Design review of the part built by this model. Coordinates are the model's own, in mm. A direction names the side the tool comes from. Round coordinates to 2 decimals unless told otherwise and drop trailing zeros. Order: outer loops, then holes, each group sorted by start corner. A loop starts at its lowest first (then second) coordinate and runs counter-clockwise, first axis right, second up. Notation, with made-up numbers: (-3.5, 43.5) - (31.5, 43.5) arc R26 cw to (31.5, 71.5) - close; hole circle Ø10 at (81, 30.5). An arc over 180 degrees is marked (long way). Write item = value, one per line.
from build123d import *

# Parameters (mm, degrees)
SKETCH1_R           = 86.36
SKETCH1_R_2         = 1.7859375
BOSS_EXTRUDE1_DEPTH = 6.35
SKETCH2_W           = 69.85
SKETCH2_H           = 114.3
CUT_EXTRUDE1_DEPTH  = 123.296450071


with BuildPart() as part:
    # Sketch1 → Boss-Extrude1 (new body)
    with BuildSketch(Plane.XY):
        Circle(SKETCH1_R)
        with Locations((0, 79.375)):
            Circle(SKETCH1_R_2, mode=Mode.SUBTRACT)
        with Locations((79.375, 0)):
            Circle(SKETCH1_R_2, mode=Mode.SUBTRACT)
        with Locations((0, -79.375)):
            Circle(SKETCH1_R_2, mode=Mode.SUBTRACT)
        with Locations((-79.375, 0)):
            Circle(SKETCH1_R_2, mode=Mode.SUBTRACT)
    extrude(amount=BOSS_EXTRUDE1_DEPTH)

    # Sketch2 → Cut-Extrude1 (cut, through all)
    with BuildSketch(Plane(origin=(0, 0, 0), x_dir=(-1, 0, 0), z_dir=(0, 0, -1))):
        Rectangle(SKETCH2_W, SKETCH2_H)
    extrude(amount=-CUT_EXTRUDE1_DEPTH, mode=Mode.SUBTRACT)


solid = part.part
1) We need section B-B on z = 1.5. Write out the cut boundary in (x, y) (3 decimals).
Findings:
outline = circle Ø172.72 at (0, 0); hole circle Ø3.572 at (-79.375, 0); hole (-34.925, -57.15) - (34.925, -57.15) - (34.925, 57.15) - (-34.925, 57.15) - close; hole circle Ø3.572 at (0, -79.375); hole circle Ø3.572 at (0, 79.375); hole circle Ø3.572 at (79.375, 0)
2) The part is to be moulded in two halves that separate along Y. For faces 1 (the cylindrical face through (-63.65, 58.37, 3.13)), 2 (the flat face through (37, 1, 6.35)), 3 (the flat face through (0, 57.15, 3)), say which applies: released by +Y, released by -Y, zero draft, split by the parting line, or undercut.
Findings:
face_1 = split by the parting line
face_2 = zero draft
face_3 = undercut
3) We need section C-C on y = -49. Write out the cut boundary in (x, z) (3 decimals).
Findings:
outline = (-71.113, 0) - (-34.925, 0) - (-34.925, 6.35) - (-71.113, 6.35) - close; (34.925, 0) - (71.113, 0) - (71.113, 6.35) - (34.925, 6.35) - close
4) We need section A-A on x = -9. Write out the cut boundary in (y, z), and give its area (3 significant figures).
Findings:
outline = (-85.89, 0) - (-57.15, 0) - (-57.15, 6.35) - (-85.89, 6.35) - close; (57.15, 0) - (85.89, 0) - (85.89, 6.35) - (57.15, 6.35) - close
area = 365 mm^2
5) For faces 4 (the flat face through (-34.925, -1, 3)), 5 (the flat face through (37, 1, 0)), list the 3-axis set-ups (+Z, -Z, +X, -X, +Y, -Y) from which the entire face can be reached by the end or side of a thin tool; tool diameter is ignored.
Findings:
face_4 = +Z, -Z
face_5 = -Z, +X, -X, +Y, -Y
6) To check wall thickness, follow L1, parallel to Y at x = 0, z = 5; L2, parallel to X at y = 44, z = 3.25 (1 decimal); L3, parallel to X at y = -18, z = 5.5 (3 decimals). State the ranges of each line that lie inside material, in increasing order. Write a range as from..to.
Findings:
L1 = -86.36..-81.16, -77.59..-57.15, 57.15..77.59, 81.16..86.36
L2 = -74.3..-34.9, 34.9..74.3
L3 = -84.463..-34.925, 34.925..84.463
7) Clearance check with flat-ended pins moving along their axes: pin 1 Ø1.5 at (x, y) = (58.5, 55.5) entering from -Z; pin 2 Ø3 at (y, z) = (26, 2.5) entering from +X; pin 3 Ø3 at (y, z) = (-17.5, 3.5) entering from -X; pin 4 Ø1.9 at (x, z) = (-2.5, 4) entering from -Y. State where each tip first meets the part, or that it passes through.
Findings:
pin_1 = 0
pin_2 = 82.81
pin_3 = -84.86
pin_4 = -86.35
8) We need section D-D on x = -38.5. Write out the cut boundary in (y, z), and give its area (3 significant figures).
Findings:
outline = (-77.3, 0) - (77.3, 0) - (77.3, 6.35) - (-77.3, 6.35) - close
area = 982 mm^2
